Could you check a few things on this model? Use its own coordinates, in mm. Face numbers are marked on the shaded views. A direction names the side the tool comes from. Round coordinates to 2 decimals unless told otherwise and drop trailing zeros. Loops run counter-clockwise (first coordinate to the right, second up) from the corner with the lowest first, then second, coordinate; pieces in that order, holes last. Notation, with made-up numbers: (-13, 55) -> (9, 55) arc R35 ccw to (9, 90) -> close; hole circle Ø10 at (-23.5, 55). An arc over 180 degrees is marked (long way). Put each result on its own line as item: value. Start each with the question number.
1. Imagine slicing it at C-C, the plane z = 0.25. Please give me the cut outline in (x, y), and give its area (3 significant figures).
2. Imagine slicing it at B-B, the plane y = 13.5. Please give me the cut outline in (x, z), and give its area (3 significant figures).
3. Which directions (+Z, -Z, +X, -X, +Y, -Y) give clear straight access to the entire face, cutting with the end or side of a thin tool? Please do the marked faces 1 and 2.
4. I need wall thicknesses on line 1 (Z direction, x = -0.75, y = 11); line 2 (X direction, y = 7.5, z = 0.25); line 3 (X direction, y = 11.25, z = 1.75). Which ranges of each line are inside material? Lowest first, please. Write a range as [from, to].
5. Imagine slicing it at A-A, the plane z = 2.75. Please give me the cut outline in (x, y).
6. If we mould it in two halves opening along Z, with no side actions, what happens to the marked faces 3, 4, 5 and 6? For each: pulls with the +Z half, pulls with the -Z half, needs draft (parallel to the pull), parting line crosses it, or undercut.
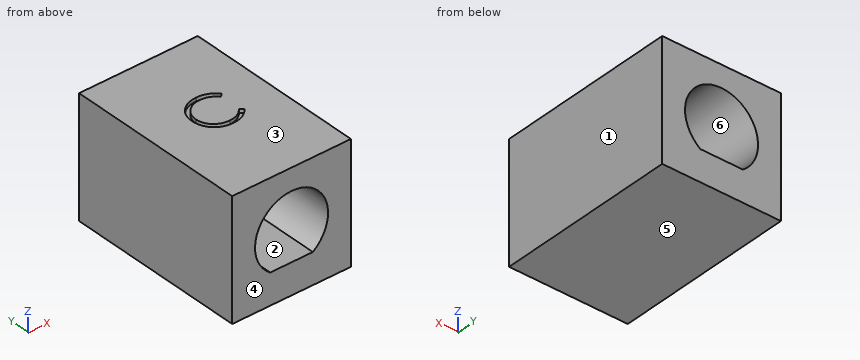
```python
from build123d import *

# Parameters (mm, degrees)
SKETCH1_W           = 9.84142284
SKETCH1_H           = 9.84142284
BOSS_EXTRUDE1_DEPTH = 15
CUT_EXTRUDE1_DEPTH  = 0.3


with BuildPart() as part:
    # Sketch1 → Boss-Extrude1 (new body)
    with BuildSketch(Plane(origin=(0, 0, 0), x_dir=(1, 0, 0), z_dir=(0, 1, 0))):
        Rectangle(SKETCH1_W, SKETCH1_H)
        with BuildLine():
            Line((-1.765045048, 2.369444822), (1.765045048, 2.369444822))
            ThreePointArc((1.765045048, 2.369444822), (0, -3.118257941), (-1.765045048, 2.369444822))
        make_face(mode=Mode.SUBTRACT)
    extrude(amount=BOSS_EXTRUDE1_DEPTH)

    # Sketch2 → Cut-Extrude1 (cut)
    with BuildSketch(Plane.XY.offset(4.92071142)):
        with BuildLine():
            Line((1.934406803, 9.11261109), (1.659567059, 8.902274552))
            add(Edge.make_bspline(
                [(1.659567059, 8.902274552), (1.639961171, 8.925640522), (1.601013724, 8.972057437), (1.538354521, 9.037236982), (1.473052878, 9.098302243), (1.405133757, 9.155544123), (1.333374638, 9.206960889), (1.259513839, 9.255231992), (1.182315794, 9.29849973), (1.075564059, 9.350962716), (0.935916211, 9.405708871), (0.760121372, 9.451612102), (0.576610273, 9.480833278), (0.451412674, 9.483998119), (0.387732123, 9.485607885)],
                knots=[0, 0, 0, 0, 9.1485e-05, 0.000181737, 0.000271024, 0.000359627, 0.000447979, 0.000535687, 0.000624217, 0.000713268, 0.000892422, 0.00107303, 0.001257466, 0.001448389, 0.001448389, 0.001448389, 0.001448389], degree=3))
            add(Edge.make_bspline(
                [(0.387732123, 9.485607885), (0.352648824, 9.485203923), (0.282807831, 9.484399747), (0.179159358, 9.473790622), (0.077446307, 9.458879412), (-0.02226516, 9.436754088), (-0.119848118, 9.408781469), (-0.21594052, 9.375356055), (-0.30915112, 9.334001215), (-0.400769358, 9.288292956), (-0.488548569, 9.236665511), (-0.571603617, 9.180352159), (-0.649631585, 9.119983062), (-0.722694197, 9.055331956), (-0.790866145, 8.986689996), (-0.853653456, 8.913325654), (-0.910838867, 8.83547348), (-0.963555892, 8.754160073), (-1.010768625, 8.669622281), (-1.050298504, 8.581547211), (-1.085303627, 8.491443108), (-1.113002869, 8.398291947), (-1.134927386, 8.302749181), (-1.150055049, 8.204558393), (-1.160543521, 8.103924714), (-1.161343697, 8.035715401), (-1.161747044, 8.001333045)],
                knots=[0, 0, 0, 0, 0.000105206, 0.000209435, 0.000312261, 0.00041348, 0.000515565, 0.000616682, 0.000718413, 0.000821258, 0.000923708, 0.001023662, 0.001122111, 0.001219464, 0.00131614, 0.001412112, 0.001508869, 0.001605718, 0.001702691, 0.001799013, 0.001895107, 0.001992482, 0.002090281, 0.00218895, 0.002290387, 0.00239349, 0.00239349, 0.00239349, 0.00239349], degree=3))
            add(Edge.make_bspline(
                [(-1.161747044, 8.001333045), (-1.160485225, 7.949601726), (-1.15800781, 7.848034141), (-1.135959476, 7.69926353), (-1.102454385, 7.556742856), (-1.052238808, 7.421363014), (-0.990319757, 7.291454656), (-0.912079146, 7.169215803), (-0.821462609, 7.052799238), (-0.717188189, 6.94495629), (-0.602782373, 6.846442565), (-0.480034462, 6.759691983), (-0.349250174, 6.687377101), (-0.211873544, 6.627201155), (-0.06684743, 6.580944427), (0.085567373, 6.548380303), (0.245039368, 6.527138123), (0.354008768, 6.525104435), (0.409466899, 6.524069424)],
                knots=[0, 0, 0, 0, 0.000155106, 0.000304531, 0.000450265, 0.000593548, 0.000736853, 0.000881182, 0.001028026, 0.001178769, 0.001330408, 0.001480379, 0.001628835, 0.001777978, 0.001929641, 0.002084627, 0.002245075, 0.00241136, 0.00241136, 0.00241136, 0.00241136], degree=3))
            add(Edge.make_bspline(
                [(0.409466899, 6.524069424), (0.470569588, 6.525758203), (0.590834297, 6.529082126), (0.767202323, 6.557241375), (0.936038089, 6.602899293), (1.097350675, 6.666797215), (1.250685321, 6.749862503), (1.396281982, 6.850560381), (1.534263552, 6.969848713), (1.617234834, 7.060931842), (1.659567059, 7.107402757)],
                knots=[0, 0, 0, 0, 0.00018322, 0.00036062, 0.000534275, 0.000707044, 0.000879893, 0.001056289, 0.001237208, 0.001425665, 0.001425665, 0.001425665, 0.001425665], degree=3))
            Line((1.659567059, 7.107402757), (1.934406803, 6.899169584))
            add(Edge.make_bspline(
                [(1.934406803, 6.899169584), (1.912288693, 6.870631132), (1.868158417, 6.813690926), (1.7967004, 6.733419216), (1.721423103, 6.65791518), (1.641767393, 6.587787559), (1.558649601, 6.521633094), (1.470577289, 6.461331262), (1.378708257, 6.406040378), (1.283353778, 6.355413454), (1.184615165, 6.310496207), (1.08261073, 6.272042439), (0.977780154, 6.238917549), (0.870118646, 6.211665612), (0.759402889, 6.190394529), (0.646032415, 6.176174854), (0.52976254, 6.166432939), (0.451321119, 6.165545024), (0.411570264, 6.165095065)],
                knots=[0, 0, 0, 0, 0.000108293, 0.000216068, 0.000322162, 0.000427957, 0.000534281, 0.00064066, 0.000747915, 0.000855806, 0.000964371, 0.001073102, 0.001182643, 0.001294024, 0.001406092, 0.001520624, 0.001636667, 0.001755891, 0.001755891, 0.001755891, 0.001755891], degree=3))
            add(Edge.make_bspline(
                [(0.411570264, 6.165095065), (0.373926597, 6.165357057), (0.299490907, 6.165875115), (0.189592155, 6.174267282), (0.082602575, 6.185717019), (-0.021172051, 6.20295715), (-0.122298026, 6.22330149), (-0.219858611, 6.250572747), (-0.314813821, 6.281121914), (-0.406782162, 6.3170269), (-0.495841862, 6.357543083), (-0.581705673, 6.403334642), (-0.664334105, 6.454016507), (-0.744539526, 6.508471517), (-0.82113711, 6.568448819), (-0.894790635, 6.633115453), (-0.965913112, 6.702253464), (-1.009915797, 6.752108317), (-1.032039512, 6.777174392)],
                knots=[0, 0, 0, 0, 0.0001129, 0.000223246, 0.000330481, 0.000435603, 0.000538732, 0.000639764, 0.000739316, 0.000837878, 0.000935767, 0.001032686, 0.001129604, 0.00122645, 0.001323362, 0.001421241, 0.001520399, 0.001620667, 0.001620667, 0.001620667, 0.001620667], degree=3))
            add(Edge.make_bspline(
                [(-1.032039512, 6.777174392), (-1.067475155, 6.82071558), (-1.137918632, 6.907272291), (-1.228044315, 7.047558272), (-1.305191871, 7.194026481), (-1.367567791, 7.34744641), (-1.416330525, 7.507473797), (-1.45011172, 7.674189311), (-1.472063324, 7.847437254), (-1.474573613, 7.965274042), (-1.475849608, 8.025171186)],
                knots=[0, 0, 0, 0, 0.000168306, 0.00033458, 0.000499224, 0.000664315, 0.00083066, 0.00100034, 0.001174094, 0.001353718, 0.001353718, 0.001353718, 0.001353718], degree=3))
            add(Edge.make_bspline(
                [(-1.475849608, 8.025171186), (-1.474294414, 8.08812664), (-1.471234668, 8.211987565), (-1.445238872, 8.393761518), (-1.403420076, 8.567912917), (-1.344023188, 8.734116661), (-1.268717836, 8.893246942), (-1.175691223, 9.044088146), (-1.06602408, 9.187604946), (-0.940576513, 9.321619697), (-0.803009177, 9.44415905), (-0.655690363, 9.551965254), (-0.498908416, 9.64168277), (-0.334390565, 9.716678932), (-0.160904883, 9.774323395), (0.021178486, 9.814676582), (0.211517401, 9.839793698), (0.341379826, 9.842968906), (0.407363533, 9.844582244)],
                knots=[0, 0, 0, 0, 0.000188789, 0.000371431, 0.000549644, 0.000725278, 0.00089996, 0.001076844, 0.001255917, 0.001440951, 0.001626689, 0.001807878, 0.001987546, 0.002167657, 0.002349462, 0.002534866, 0.002726448, 0.002924344, 0.002924344, 0.002924344, 0.002924344], degree=3))
            add(Edge.make_bspline(
                [(0.407363533, 9.844582244), (0.447578005, 9.844100106), (0.527178503, 9.843145762), (0.644931155, 9.83383962), (0.759573482, 9.818326014), (0.871184464, 9.797209944), (0.98030708, 9.771002622), (1.086107321, 9.736862324), (1.189206008, 9.697825793), (1.288952916, 9.652867327), (1.384869466, 9.602400585), (1.476925785, 9.546984962), (1.564390643, 9.486689156), (1.647879492, 9.422025981), (1.725995703, 9.351627422), (1.800957181, 9.277429826), (1.87021826, 9.197296001), (1.912971455, 9.140891068), (1.934406803, 9.11261109)],
                knots=[0, 0, 0, 0, 0.000120626, 0.000238766, 0.000354085, 0.000467531, 0.000579423, 0.000690512, 0.000800803, 0.000910007, 0.001018518, 0.001125773, 0.001232152, 0.001337058, 0.001442329, 0.001547432, 0.001653292, 0.001759736, 0.001759736, 0.001759736, 0.001759736], degree=3))
        make_face()
    extrude(amount=-CUT_EXTRUDE1_DEPTH, mode=Mode.SUBTRACT)


solid = part.part
```
Entries:
1. outline: (-4.92, 0) -> (-3.02, 0) -> (-3.02, 15) -> (-4.92, 15) -> close; (3.02, 0) -> (4.92, 0) -> (4.92, 15) -> (3.02, 15) -> close
1. area: 56.9 mm^2
2. outline: (-4.92, -4.92) -> (4.92, -4.92) -> (4.92, 4.92) -> (-4.92, 4.92) -> close; hole (-1.77, -2.37) -> (1.77, -2.37) arc R3.03 ccw (long way) to start
2. area: 69.4 mm^2
3. face 1: +Z, -Z, +X, +Y, -Y
3. face 2: +Y, -Y
4. line 1: [-4.92, -2.37], [3.02, 4.92]
4. line 2: [-4.92, -3.02], [3.02, 4.92]
4. line 3: [-4.92, -2.53], [2.53, 4.92]
5. outline: (-4.92, 0) -> (-1.45, 0) -> (-1.45, 15) -> (-4.92, 15) -> close; (1.45, 0) -> (4.92, 0) -> (4.92, 15) -> (1.45, 15) -> close
6. face 3: pulls with the +Z half
6. face 4: needs draft
6. face 5: pulls with the -Z half
6. face 6: undercut
